Source: three-view drawing plus pictorial views. Frame: mm from the lowest corner of the part. Round coordinates to 2 decimals unless told otherwise and drop trailing zeros. Order: outer loops, then holes, each group sorted by start corner. A loop starts at its lowest first (then second) coordinate and runs counter-clockwise, first axis right, second up. Notation, with made-up numbers: (-12.75, 11) -> (23.25, 11) arc R28 cw to (23.25, 30) -> close; hole circle Ø2 at (78, 61). An arc over 180 degrees is marked (long way). Use a Markdown table: item, result.
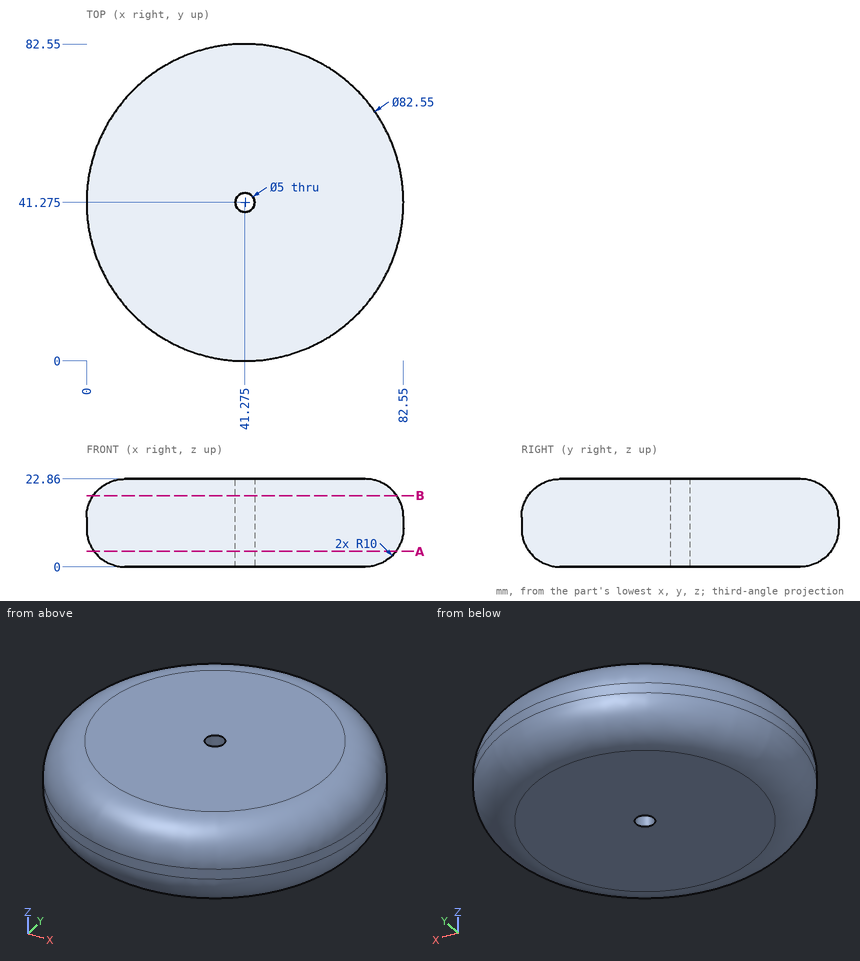
1) Cut plane B-B on z = 18.5. Return loops of the section in (x, y) (1 decimal), and give its area (3 significant figures).
Results found:
| item | result |
|---|---|
| outline | circle Ø79.1 at (41.3, 41.3); hole circle Ø5 at (41.3, 41.3) |
| area | 4,890 mm² |
2) Pin query (flat end, axial travel): pin 1 Ø5 at (y, z) = (19, 18) entering from +X; pin 2 Ø5 at (x, y) = (67.5, 18.5) entering from +Z; pin 3 Ø6 at (x, z) = (43.5, 11.5) entering from -Y. Return the tip coordinate at first contact, or that it passes through.
Results found:
| item | result |
|---|---|
| pin 1 | stops at x = 76.44 |
| pin 2 | stops at z = 22.81 |
| pin 3 | stops at y = 0 |
3) Line query: L1, parallel to X at y = 20, z = 14.25; L2, parallel to Z at x = 4, y = 25.5; L3, parallel to Y at x = 26, z = 10.5. Output: solid intervals per line, ascending. Write a range as [from, to].
Results found:
| item | result |
|---|---|
| L1 | x = [6.02, 76.53] |
| L2 | z = [6.08, 16.78] |
| L3 | y = [2.93, 79.62] |
4) Cut plane A-A on z = 4. Return loops of the section in (x, y) (3 decimals).
Results found:
| item | result |
|---|---|
| outline | circle Ø78.55 at (41.275, 41.275); hole circle Ø5 at (41.275, 41.275) |
